```python
from build123d import *

# Parameters (mm, degrees)
BOSS_EXTRUDE1_DEPTH         = 4.5
TAP_DRILL_FOR_M4X0_7_TAP1_D = 3.3


with BuildPart() as part:
    # Sketch1 → Boss-Extrude1 (new body, symmetric)
    with BuildSketch(Plane(origin=(0, 0, 0), x_dir=(1, 0, 0), z_dir=(0, 1, 0))):
        with BuildLine():
            Line((-27.5, 0), (-17.5, 0))
            ThreePointArc((-17.5, 0), (0, 17.5), (17.5, 0))
            Line((17.5, 0), (27.5, 0))
            ThreePointArc((27.5, 0), (0, 27.5), (-27.5, 0))
        make_face()
    extrude(amount=BOSS_EXTRUDE1_DEPTH, both=True)

    # Tap Drill for M4x0.7 Tap1 (through all)
    with Locations(Plane(origin=(22.5, 0, 0), x_dir=(1, 0, 0), z_dir=(0, 0, 1))):
        with Locations((0, 0), (-45, 0)):
            Hole(TAP_DRILL_FOR_M4X0_7_TAP1_D / 2)


solid = part.part
```
For this review, take the finished solid that the model builds, in its own axes (mm). Coordinates: 2 decimals unless noted, no trailing zeros. Write each loop counter-clockwise with the first axis right and the second up, starting at its lowest first coordinate (ties: lowest second). Pieces come first, ordered by that corner, then holes. Notation, with made-up numbers: (8, 44.25) - (28, 44.25) arc R15 ccw to (28, 64.25) - close; hole circle Ø9 at (-10, -39). An arc over 180 degrees is marked (long way). Put each result on its own line as item: value.
1. Add section B-B, the plane y = 0. Give the boundary of the cut face in (x, z), then the cut area to 3 significant figures.
Values found:
outline: (-27.5, 0) arc R27.5 ccw to (-24.15, -13.15) - (-24.15, 0) - close; (-20.85, -17.93) arc R27.5 ccw to (20.85, -17.93) - (20.85, 0) - (17.5, 0) arc R17.5 cw to (-17.5, 0) - (-20.85, 0) - close; (24.15, -13.15) arc R27.5 ccw to (27.5, 0) - (24.15, 0) - close
area: 603 mm²
2. Add section D-D, the plane x = -22.5. Give the boundary of the cut face in (y, z), then the cut area to 3 significant figures.
Values found:
outline: (-4.5, -15.81) - (-1.65, -15.81) - (-1.65, 0) - (-4.5, 0) - close; (1.65, -15.81) - (4.5, -15.81) - (4.5, 0) - (1.65, 0) - close
area: 90.1 mm²
3. Wall thickness on probe 1 along Y at (x, z) = (-22.5, -8.5); probe 2 along X at (y, z) = (0, -3.75); probe 3 along X at (y, z) = (-2.25, -7.5): over which ranges is each line inside the solid? List them lowest first.
Values found:
probe 1: -4.5 to -1.65, 1.65 to 4.5
probe 2: -27.24 to -24.15, -20.85 to -17.09, 17.09 to 20.85, 24.15 to 27.24
probe 3: -26.46 to -15.81, 15.81 to 26.46
4. Add section A-A, the plane z = -2.5. Give the boundary of the cut face in (x, y), then the cut area to 3 significant figures.
Values found:
outline: (-27.39, -4.5) - (-17.32, -4.5) - (-17.32, 4.5) - (-27.39, 4.5) - close; (17.32, -4.5) - (27.39, -4.5) - (27.39, 4.5) - (17.32, 4.5) - close; hole circle Ø3.3 at (-22.5, 0); hole circle Ø3.3 at (22.5, 0)
area: 164 mm²
5. Mouldability with a two-part tool opening along Y and no side actions: class faces 1 (the flat face through (0, 4.5, -20)), 2 (the flat face through (-23, 2, 0)), 3 (the cylindrical face through (20.926, 0.496, -7.099)) as released by +Y, released by -Y, zero draft, split by the parting line, or undercut.
Values found:
face 1: released by +Y
face 2: zero draft
face 3: undercut
6. Add section C-C, the plane z = -16.5. Give the boundary of the cut face in (x, y), then the cut area to 3 significant figures.
Values found:
outline: (-22, -4.5) - (-5.83, -4.5) - (-5.83, 4.5) - (-22, 4.5) - (-22, 1.57) arc R1.65 cw to (-22, -1.57) - close; (5.83, -4.5) - (22, -4.5) - (22, -1.57) arc R1.65 cw to (22, 1.57) - (22, 4.5) - (5.83, 4.5) - close
area: 286 mm²
7. For pin 1 (1 mm diameter, centred on y = 1.5, z = -16.5, fed in from -X); pin 2 (2.5 mm diameter, centred on x = 22.5, y = 0, fed in from +Z); pin 3 (2 mm diameter, centred on x = 18, y = -3, fed in from -Z); pin 4 (8 mm diameter, centred on x = -12.5, z = -10.5, fed in from +Y), all flat-tipped, find the tip position at first contact; note any pin that passes through.
Values found:
pin 1: x = -22.35
pin 2: through
pin 3: z = -21.62
pin 4: y = 4.5
